For this review, take the finished solid that the model builds, in its own axes (mm). A direction names the side the tool comes from. Round coordinates to 2 decimals unless told otherwise and drop trailing zeros. Loops run counter-clockwise (first coordinate to the right, second up) from the corner with the lowest first, then second, coordinate; pieces in that order, holes last.
1) Wall thickness on L1, parallel to Y at x = 22, z = 65; L2, parallel to X at y = -4, z = 50.5: over which ranges is each line inside the solid? List them lowest first.
2) Mouldability with a two-part tool opening along Y and no side actions: class faces 3 (the flat face through (1, 63.5, 44)), 4 (the flat face through (-88.9, -1, 44)), 5 (the flat face through (-1, 44.45, 44)) as pulls with the +Y half, pulls with the -Y half, needs draft (parallel to the pull), parting line crosses it, or undercut.
3) Take a section at B-B (z = 66). State the section outline as (x, y) points.
4) Take a section at A-A (y = -1). State the section outline as (x, z) points.
5) Tool access review of faces 1 (the flat face through (-69.85, -1, 44)), 2 (the flat face through (-1, -56, 0)): name each direction out of +Z, -Z, +X, -X, +Y, -Y from which nothing blocks a thin tool from reaching the whole face with its end or side.
6) Take a section at C-C (x = 2). State the section outline as (y, z) points.
```python
from build123d import *

# Parameters (mm, degrees)
F1_DEPTH = 88.9
F0_W     = 19.05
F0_H     = 88.9
F2_DEPTH = 88.9


with BuildPart() as f1:
    # F0 (on Top) → F1 (new body)
    with BuildSketch(Plane.XY):
        Polygon((88.9, 63.5), (-88.9, 63.5), (-88.9, 44.45), (-69.85, 44.45), (69.85, 44.45), (88.9, 44.45), align=None)
        Polygon((-69.85, -44.45), (-88.9, -44.45), (-88.9, -63.5), (88.9, -63.5), (88.9, -44.45), (69.85, -44.45), align=None)
    extrude(amount=F1_DEPTH)

    # F0 (on Top) → F2 (join)
    with BuildSketch(Plane.XY):
        with Locations((-79.375, 0)):
            Rectangle(F0_W, F0_H)
        with Locations((79.375, 0)):
            Rectangle(F0_W, F0_H)
    extrude(amount=F2_DEPTH)


solid = f1.part
```
Response:
1. L1: y = -63.5 to -44.45, 44.45 to 63.5
1. L2: x = -88.9 to -69.85, 69.85 to 88.9
2. face 3: pulls with the +Y half
2. face 4: needs draft
2. face 5: undercut
3. outline: (-88.9, -63.5) - (88.9, -63.5) - (88.9, 63.5) - (-88.9, 63.5) - close; hole (-69.85, -44.45) - (69.85, -44.45) - (69.85, 44.45) - (-69.85, 44.45) - close
4. outline: (-88.9, 0) - (-69.85, 0) - (-69.85, 88.9) - (-88.9, 88.9) - close; (69.85, 0) - (88.9, 0) - (88.9, 88.9) - (69.85, 88.9) - close
5. face 1: +Z, -Z
5. face 2: -Z, +X, -X, +Y, -Y
6. outline: (-63.5, 0) - (-44.45, 0) - (-44.45, 88.9) - (-63.5, 88.9) - close; (44.45, 0) - (63.5, 0) - (63.5, 88.9) - (44.45, 88.9) - close
